Check sheet for the drawn part. Datum: minimum x, y, z corner. Units: mm. Round coordinates to 2 decimals unless told otherwise and drop trailing zeros. Write each loop counter-clockwise with the first axis right and the second up, starting at its lowest first coordinate (ties: lowest second). Pieces come first, ordered by that corner, then holes.
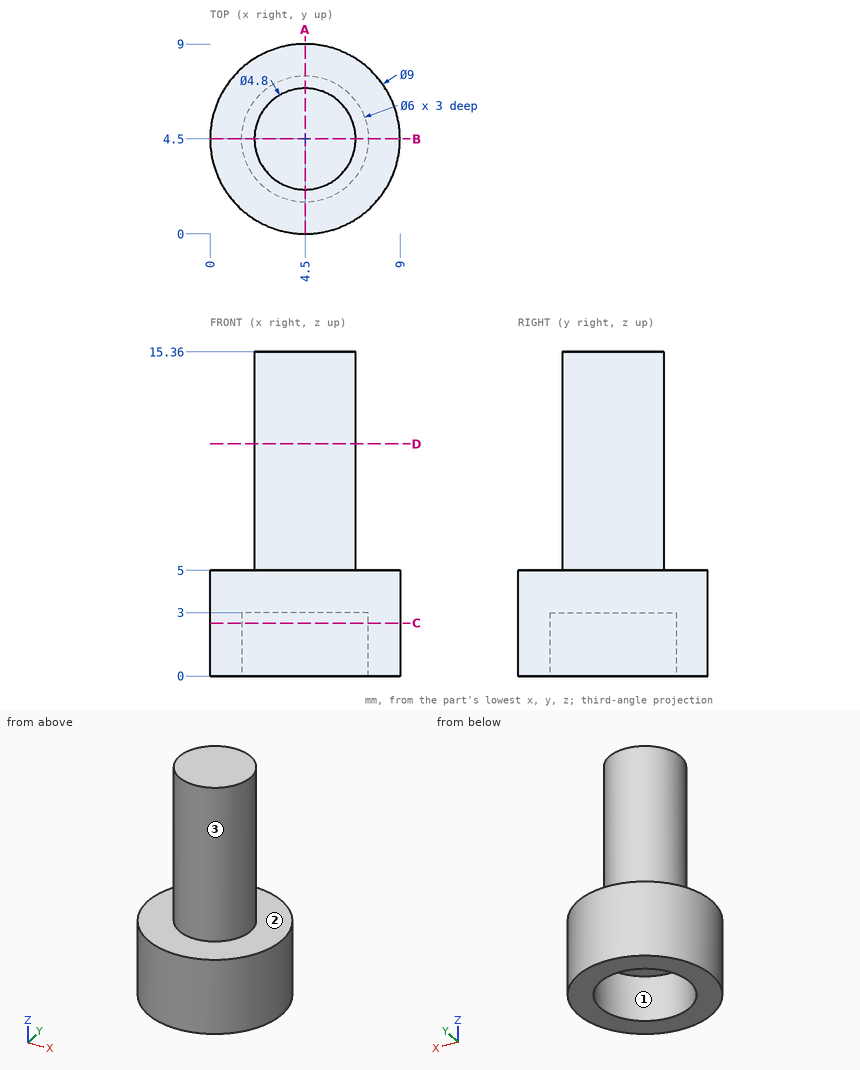
Q1. Depth check by flat-ended pin: P1, Ø2, axis at x = 1.5, z = 4.5, coming from the -Y side; P2, Ø2, axis at y = 7.5, z = 5, coming from the -X side; P3, Ø3, axis at x = 7.5, z = 9, coming from the -Y side; P4, Ø2, axis at x = 1.5, y = 1, coming from the -Z side. Enter the tip coordinate at first touch or a pass-through.
Recorded:
P1: stops at y = 0.47
P2: stops at x = 0.47
P3: stops at y = 2.63
P4: stops at z = 0
Q2. Sectioned sample at C-C (z = 2.5). Enter the section's corners in (x, y), plus the area to 3 significant figures.
Recorded:
outline: circle Ø9 at (4.5, 4.5); hole circle Ø6 at (4.5, 4.5)
area: 35.3 mm2
Q3. Material ranges on line 1 along Y through (x, z) = (4.5, 1.75); line 2 along Z through (x, y) = (5.5, 2.75); line 3 along Z through (x, y) = (4.25, 0.5), recorded low to high.
Recorded:
line 1: y = 0 to 1.5, 7.5 to 9
line 2: z = 3 to 15.36
line 3: z = 0 to 5
Q4. Sectioned sample at A-A (x = 4.5). Enter the section's corners in (y, z), plus the area to 3 significant figures.
Recorded:
outline: (0, 0) - (1.5, 0) - (1.5, 3) - (7.5, 3) - (7.5, 0) - (9, 0) - (9, 5) - (6.9, 5) - (6.9, 15.36) - (2.1, 15.36) - (2.1, 5) - (0, 5) - close
area: 76.7 mm2
Q5. Sectioned sample at D-D (z = 11). Enter the section's corners in (x, y).
Recorded:
outline: circle Ø4.8 at (4.5, 4.5)
Q6. Release check for a two-part mould opening along Y. For the marked faces 1, 2 and 3 record: released by +Y, released by -Y, zero draft, split by the parting line, or undercut.
Recorded:
face 1: undercut
face 2: zero draft
face 3: split by the parting line
